CAD build for the part. Positions are in the model's coordinates, mm. Face numbers are marked on the shaded views. A direction names the side the tool comes from. Round coordinates to 2 decimals unless told otherwise and drop trailing zeros. Loops run counter-clockwise (first coordinate to the right, second up) from the corner with the lowest first, then second, coordinate; pieces in that order, holes last. Notation, with made-up numbers: M 33,72.25 L 62,72.25 A21 ccw 62,81.25 Z; hole C 4.25,15 d8. An arc over 180 degrees is marked long. Use a Markdown table: item, result. Add a question column.
(1) Band-saw the part on C-C, the plane x = 32.5. Write the cut outline in (y, z).
(2) Which spindle directions (+Z, -Z, +X, -X, +Y, -Y) get a long thin tool onto all of the face, cutting with end or side? Do the marked faces 1 and 2. Say none if no direction does.
(3) Wall check: L1, parallel to Z at x = 21, y = 0; L2, parallel to Z at x = 4.25, y = 0; L3, parallel to Y at x = 20, z = -25. Give the ranges that are in metal, low to high.
(4) Band-saw the part on A-A, the plane y = 0. Write the cut outline in (x, z).
(5) Flat gauge pins, fed straight in: P1, Ø11, axis at y = 0, z = -25.4, coming from the +X side; P2, Ø19, axis at y = 22.5, z = 7.5, coming from the -X side; P3, Ø9, axis at x = 11, z = -3, coming from the +Y side. Where does each tip first touch, or does it go through?
(6) Band-saw the part on B-B, the plane z = 25.4. Write the cut outline in (x, y).
(7) Band-saw the part on D-D, the plane z = -30. Write the cut outline in (x, y), and give its area (3 significant figures).
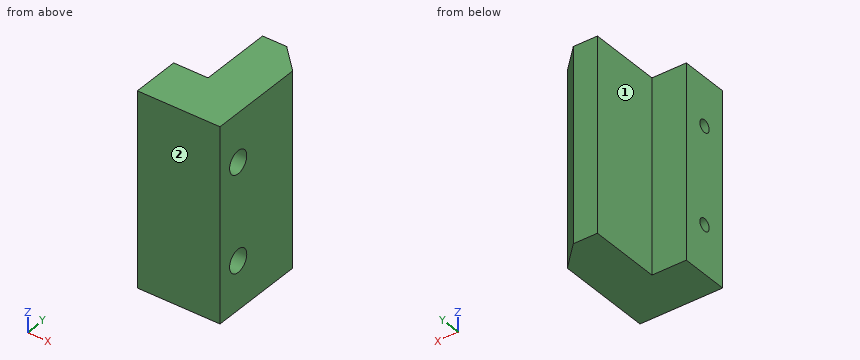
from build123d import *

# Parameters (mm, degrees)
BOSS_EXTRUDE1_DEPTH = 50.8
SKETCH2_R           = 3.25
CUT_EXTRUDE1_DEPTH  = 84.985296332
SKETCH3_R           = 6
CUT_EXTRUDE2_DEPTH  = 33.5


with BuildPart() as part:
    # Sketch1 → Boss-Extrude1 (new, symmetric)
    with BuildSketch(Plane.XY):
        Polygon((43.5, 38.1), (30.8, 50.8), (18.1, 50.8), (18.1, 12.7), (0, 12.7), (0, -12.7), (43.5, -12.7), align=None)
    extrude(amount=BOSS_EXTRUDE1_DEPTH, both=True)

    # Sketch2 → Cut-Extrude1 (cut, through all)
    with BuildSketch(Plane(origin=(43.5, 0, 0), x_dir=(0, 0, -1), z_dir=(1, 0, 0))):
        with Locations(Location((-25.4, 0, 0), (0, 0, 90))):
            Circle(SKETCH2_R)
        with Locations(Location((25.4, 0, 0), (0, 0, 90))):
            Circle(SKETCH2_R)
    extrude(amount=-CUT_EXTRUDE1_DEPTH, mode=Mode.SUBTRACT)

    # Sketch3 → Cut-Extrude2 (cut)
    with BuildSketch(Plane(origin=(43.5, 0, 0), x_dir=(0, 0, -1), z_dir=(1, 0, 0))):
        with Locations(Location((-25.4, 0, 0), (0, 0, 90))):
            Circle(SKETCH3_R)
        with Locations(Location((25.4, 0, 0), (0, 0, 90))):
            Circle(SKETCH3_R)
    extrude(amount=-CUT_EXTRUDE2_DEPTH, mode=Mode.SUBTRACT)


solid = part.part
Return value:
| question | item | result |
|---|---|---|
| 1 | outline | M -12.7,-50.8 L 49.1,-50.8 L 49.1,50.8 L -12.7,50.8 Z; hole C 0,-25.4 d12; hole C 0,25.4 d12 |
| 2 | face 1 | +Z, -Z, -X, +Y |
| 2 | face 2 | +Z, -Z, +X, -X, -Y |
| 3 | L1 | -50.8 to -31.4, -19.4 to 19.4, 31.4 to 50.8 |
| 3 | L2 | -50.8 to -28.65, -22.15 to 22.15, 28.65 to 50.8 |
| 3 | L3 | -12.7 to -5.99, 5.99 to 50.8 |
| 4 | outline | M 0,-50.8 L 43.5,-50.8 L 43.5,-31.4 L 10,-31.4 L 10,-28.65 L 0,-28.65 Z; M 0,-22.15 L 10,-22.15 L 10,-19.4 L 43.5,-19.4 L 43.5,19.4 L 10,19.4 L 10,22.15 L 0,22.15 Z; M 0,28.65 L 10,28.65 L 10,31.4 L 43.5,31.4 L 43.5,50.8 L 0,50.8 Z |
| 5 | P1 | x = 10 |
| 5 | P2 | x = 18.1 |
| 5 | P3 | y = 12.7 |
| 6 | outline | M 0,-12.7 L 43.5,-12.7 L 43.5,-6 L 10,-6 L 10,-3.25 L 0,-3.25 Z; M 0,3.25 L 10,3.25 L 10,6 L 43.5,6 L 43.5,38.1 L 30.8,50.8 L 18.1,50.8 L 18.1,12.7 L 0,12.7 Z |
| 7 | outline | M 0,-12.7 L 43.5,-12.7 L 43.5,-3.85 L 10,-3.85 L 10,3.85 L 43.5,3.85 L 43.5,38.1 L 30.8,50.8 L 18.1,50.8 L 18.1,12.7 L 0,12.7 Z |
| 7 | area | 1,730 mm^2 |
